For this review, take the finished solid that the model builds, in its own axes (mm). Give positions to 0.01 mm unless a question says otherwise; leave off trailing zeros. Write each loop counter-clockwise with the first axis right and the second up, starting at its lowest first coordinate (ties: lowest second). Pieces come first, ordered by that corner, then holes. Notation, with made-up numbers: (8.25, 14.25) -> (46.25, 14.25) arc R29 cw to (46.25, 42.25) -> close; hole circle Ø7 at (-8, -0.5). An arc over 180 degrees is marked (long way). Return JSON: item names as keys, results as strings.
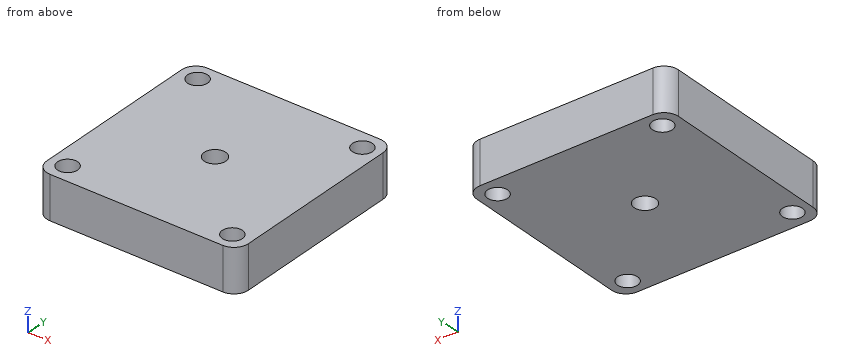
Autodesk Inventor part; units mm, degrees
ref_plane "YZ Plane" through (0, 0, 0) normal (1, 0, 0) x (0, 1, 0)
ref_plane "XZ Plane" through (0, 0, 0) normal (0, 1, 0) x (-1, 0, 0)
ref_plane "XY Plane" through (0, 0, 0) normal (0, 0, 1) x (1, 0, 0)
ref_plane "Arbeitsebene1" through (0, 0, 0) normal (0, 0, 1) x (1, 0, 0)
sketch "Skizze1" plane through (0, 0, 0) normal (0, 0, 1) x (1, 0, 0)
  line L0 (11.7109, -4.9124) -> (9.211, -4.9293)
  line L1 (9.211, -4.9293) -> (9.1974, -2.9294)
  line L2 (9.1974, -2.9294) -> (-3.8023, -3.0177)
  line L3 (-3.8023, -3.0177) -> (-3.8306, 1.1495)
  line L4 (-3.8306, 1.1495) -> (-6.8306, 1.1291)
  line L5 (-6.8306, 1.1291) -> (-6.6653, -23.2049)
  line L6 (-6.6653, -23.2049) -> (-3.6653, -23.1845)
  line L7 (-3.6653, -23.1845) -> (-3.6937, -19.0173)
  line L8 (-3.6937, -19.0173) -> (9.306, -18.929)
  line L9 (9.306, -18.929) -> (9.2925, -16.9291)
  line L10 (9.2925, -16.9291) -> (11.7924, -16.9121)
  line L11 (11.7924, -16.9121) -> (11.7109, -4.9124)
  circle A0 centre (13.7364, 0.5156) radius 1.025
  circle A1 centre (13.7676, -22.4844) radius 1.025
  circle A2 centre (-9.2323, -22.5156) radius 1.025
  circle A3 centre (-9.2636, 0.4844) radius 1.025
  line L12 (-11.8291, 0.9046) -> (-11.6661, -23.0948)
  arc A4 (-9.8428, 2.9182) -> (-11.8291, 0.9046) centre (-9.8292, 0.9182) ccw
  line L13 (14.1567, 3.0812) -> (-9.8428, 2.9182)
  arc A5 (16.1702, 1.0948) -> (14.1567, 3.0812) centre (14.1703, 1.0812) ccw
  line L14 (16.3332, -22.9046) -> (16.1702, 1.0948)
  arc A6 (14.3468, -24.9182) -> (16.3332, -22.9046) centre (14.3333, -22.9182) ccw
  line L15 (-9.6526, -25.0812) -> (14.3468, -24.9182)
  arc A7 (-11.6661, -23.0948) -> (-9.6526, -25.0812) centre (-9.6662, -23.0812) ccw
  circle A8 centre (2.252, -11) radius 7.5
  circle A9 centre (2.252, -11) radius 1.5
  circle A10 centre (-9.2323, -22.5156) radius 1.4
  circle A11 centre (13.7676, -22.4844) radius 1.4
  circle A12 centre (-9.2636, 0.4844) radius 1.4
  circle A13 centre (13.7364, 0.5156) radius 1.4
  point P0 (0, 0)
  dimension "d0" = 3
  dimension "d1" = 2.8
  dimension "d2" = 2.8
  dimension "d3" = 2.8
  dimension "d4" = 2.8
extrude "Extrusion1" add sketch "Skizze1" against normal blind 6 contours L11 L10 L9 L8 L7 L6 L5 L4 L3 L2 L1 L0 | A4 L13 A5 L14 A6 L15 A7 L12 | A8
properties part number "00_Micro_Stepper_15mm_Gearbox_counterbearing"
1. Add section A-A, the plane y = -11.5. State the section outline as (x, z) points, plus the area to 3 significant figures.
Results found:
{"outline": "(-11.74, -6) -> (0.84, -6) -> (0.84, 0) -> (-11.74, 0) -> close; (3.67, -6) -> (16.26, -6) -> (16.26, 0) -> (3.67, 0) -> close", "area": "151 mm²"}
2. To check wall thickness, follow probe 1 along X at (y, z) = (0.5, -4.55); probe 2 along Y at (x, z) = (-9.25, -5.5); probe 3 along X at (y, z) = (-21.25, -4.1). State the ranges of each line that lie inside material, in increasing order.
Results found:
{"probe 1": "x = -11.83 to -10.66, -7.86 to 12.34, 15.14 to 16.17", "probe 2": "y = -25.08 to -23.92, -21.12 to -0.92, 1.88 to 2.92", "probe 3": "x = -11.68 to -9.83, -8.63 to 13.11, 14.43 to 16.32"}
3. Add section B-B, the plane z = -2.7. State the section outline as (x, y) points.
Results found:
{"outline": "(-11.83, 0.9) -> (-11.67, -23.09) arc R2 ccw to (-9.65, -25.08) -> (14.35, -24.92) arc R2 ccw to (16.33, -22.9) -> (16.17, 1.09) arc R2 ccw to (14.16, 3.08) -> (-9.84, 2.92) arc R2 ccw to start; hole circle Ø2.8 at (-9.26, 0.48); hole circle Ø2.8 at (-9.23, -22.52); hole circle Ø3 at (2.25, -11); hole circle Ø2.8 at (13.74, 0.52); hole circle Ø2.8 at (13.77, -22.48)"}
4. For pin 1 (5 mm diameter, centred on x = 3, y = -21.5, fed in from +Z), flat-tipped, find the tip position at first contact; note if it passes through.
Results found:
{"pin 1": "stops at z = 0"}
